```python
from build123d import *

# Parameters (mm, degrees)
EXTRUDE_1_DEPTH        = 9
SKETCH_3_R             = 15
CUT_EXTRUDE_1_DEPTH    = 26.5
HOLE_WIZARD_M6_1_D     = 5
HOLE_WIZARD_M6_1_DEPTH = 17
HOLE_WIZARD_M6_1_TIP   = 1.502151548
CHAMFER_1_SIZE         = 1
SKETCH_6_W             = 1.1
SKETCH_6_H             = 0.3


with BuildPart() as part:
    # 草图1 → 旋转1 (revolve)
    with BuildSketch(Plane.XY):
        Polygon((-129, 0), (129, 0), (129, 6), (128, 7), (33, 7), (33, 10), (31, 10), (31, 7), (-128.5, 7), (-129, 6.5), align=None)
    revolve(axis=Axis((-129, 0, 0), (1, 0, 0)))

    # 草图2 → 凸台-拉伸1 (add)
    with BuildSketch(Plane.XY):
        with BuildLine():
            ThreePointArc((-108, 2.5), (-105.5, 0), (-108, -2.5))
            Line((-108, -2.5), (-123, -2.5))
            ThreePointArc((-123, -2.5), (-125.5, 0), (-123, 2.5))
            Line((-123, 2.5), (-108, 2.5))
        make_face()
        with BuildLine():
            Line((38, -2.5), (48, -2.5))
            ThreePointArc((48, -2.5), (50.5, 0), (48, 2.5))
            Line((48, 2.5), (38, 2.5))
            ThreePointArc((38, 2.5), (35.5, 0), (38, -2.5))
        make_face()
        with BuildLine():
            Line((123, 2.5), (108, 2.5))
            ThreePointArc((108, 2.5), (105.5, 0), (108, -2.5))
            Line((108, -2.5), (123, -2.5))
            ThreePointArc((123, -2.5), (125.5, 0), (123, 2.5))
        make_face()
        with BuildLine():
            Line((81, -2.5), (91, -2.5))
            ThreePointArc((91, -2.5), (93.5, 0), (91, 2.5))
            Line((91, 2.5), (81, 2.5))
            ThreePointArc((81, 2.5), (78.5, 0), (81, -2.5))
        make_face()
    extrude(amount=EXTRUDE_1_DEPTH)

    # 草图3 → 切除-拉伸1 (cut)
    with BuildSketch(Plane(origin=(129, 0, 0), x_dir=(0, 0, -1), z_dir=(1, 0, 0))):
        Circle(SKETCH_3_R)
    extrude(amount=-CUT_EXTRUDE_1_DEPTH, mode=Mode.SUBTRACT)

    # M6 螺纹孔1
    with Locations(Plane.ZY.offset(129)):
        with Locations((0, 0)):
            Hole(HOLE_WIZARD_M6_1_D / 2, depth=HOLE_WIZARD_M6_1_DEPTH)
            with Locations((0, 0, -(HOLE_WIZARD_M6_1_DEPTH + HOLE_WIZARD_M6_1_TIP / 2))):  # 118° drill point
                Cone(0, HOLE_WIZARD_M6_1_D / 2, HOLE_WIZARD_M6_1_TIP, mode=Mode.SUBTRACT)

    # 倒角1
    chamfer_1_edges = [part.edges().sort_by_distance(p)[0] for p in [
        (102.5, -7, 0),
    ]]
    chamfer(chamfer_1_edges, length=CHAMFER_1_SIZE)

    # 草图6 → 切除-旋转1 (revolve, cut)
    with BuildSketch(Plane.XY):
        with Locations((96.55, -6.85)):
            Rectangle(SKETCH_6_W, SKETCH_6_H)
    revolve(axis=Axis((0, 0, 0), (1, 0, 0)), mode=Mode.SUBTRACT)


solid = part.part
```
Build history of the part. All positions in model axes, mm. A direction names the side the tool comes from. Give positions to 0.01 mm unless a question says otherwise; leave off trailing zeros. Loops run counter-clockwise (first coordinate to the right, second up) from the corner with the lowest first, then second, coordinate; pieces in that order, holes last.
1) Band-saw the part on A-A on x = 40. List the corners of the cut face in (y, z).
Values follow:
outline: (-2.5, 6.54) arc R7 ccw (long way) to (2.5, 6.54) - (2.5, 9) - (-2.5, 9) - close
2) Two-plate mould, pull along X, no slides. Class faces 1 (the face through (-110.759, -0.424, -0.094)), 2 (the face through (96.558, 6.694, -0.295)), 3 (the face through (102.5, 0, 0)), 4 (the face through (-115, 0, 9)): released by +X, released by -X, zero draft, split by the parting line, or undercut.
Values follow:
face 1: released by -X
face 2: undercut
face 3: released by +X
face 4: zero draft
3) Band-saw the part on B-B on x = -91. List the corners of the cut face in (y, z), then the cut area to 3 significant figures.
Values follow:
outline: circle Ø14 at (0, 0)
area: 154 mm2
4) Drop flat-ended pins along their axis: P1, Ø2.5, axis at x = 87, z = 8, coming from the +Y side; P2, Ø0.7, axis at x = -115, z = 8.5, coming from the -Y side; P3, Ø8, axis at x = 5, y = 5.5, coming from the -Z side. Give the stop position or say it passes through.
Values follow:
P1: stops at y = 2.5
P2: stops at y = -2.5
P3: stops at z = -6.84
5) Probe line 1 along Z through (x, y) = (-121.5, 0); line 2 along Z through (x, y) = (-113.5, 0.5); line 3 along X through (y, z) = (-6.75, 6.25). List the from-to ranges inside material, lowest first.
Values follow:
line 1: z = -7 to -2.5, 2.5 to 9
line 2: z = -6.98 to -2.45, 2.45 to 9
line 3: x = 31 to 33
6) 3-axis set-ups, long thin cutter, end or side, ignore diameter. For faces 5 (the face through (-120.38, -2.44, 0.54)), 6 (the face through (-129, 3, 0)), 7 (the face through (31.99, -2.17, -9.76)), 8 (the face through (43, 0, 9)), 9 (the face through (99.269, 6.466, -2.681)): which of +Z, -Z, +X, -X, +Y, -Y reach the whole face in a straight line?
Values follow:
face 5: -X
face 6: +Z, -Z, -X, +Y, -Y
face 7: +X, -X
face 8: +Z, +X, +Y, -Y
face 9: +X
